For this review, take the finished solid that the model builds, in its own axes (mm). Face numbers are marked on the shaded views. A direction names the side the tool comes from. Coordinates: 2 decimals unless noted, no trailing zeros. Loops run counter-clockwise (first coordinate to the right, second up) from the corner with the lowest first, then second, coordinate; pieces in that order, holes last. Notation, with made-up numbers: (50.25, 5.5) - (54.25, 5.5) arc R22 ccw to (54.25, 35.5) - close; hole circle Ø7 at (86, 18.25). An arc over 180 degrees is marked (long way). Answer as a JSON object with one key per item and string values. Group by question number.
Item 1: We need section B-B (x = -16). Give the boundary of the cut face in (y, z).
Item 2: Clearance check with flat-ended pins moving along their axes: pin 1 (1.5 mm diameter, centred on y = 3.5, z = 4, fed in from -X); pin 2 (6.5 mm diameter, centred on x = 3.5, z = -4.5, fed in from +Y); pin 3 (3 mm diameter, centred on x = -2, z = 9.5, fed in from +Y); pin 4 (4 mm diameter, centred on x = 10.5, y = 5, fed in from +Z). State where each tip first meets the part, or that it passes through.
Item 3: We need section A-A (y = 4.5). Give the boundary of the cut face in (x, z), then the cut area to 3 significant figures.
Item 4: To check wall thickness, follow line 1 (X direction, y = 5, z = 8); line 2 (Z direction, x = 15, y = 3.25); line 3 (X direction, y = 6.25, z = -3). State the ranges of each line that lie inside material, in increasing order.
Item 5: We need section D-D (z = 8). Give the boundary of the cut face in (x, y), then the cut area to 3 significant figures.
Item 6: We need section C-C (z = 1). Give the boundary of the cut face in (x, y), then the cut area to 3 significant figures.
Item 7: Mouldability with a two-part tool opening along X and no side actions: class the marked faces 5, 6 and 7 as released by +X, released by -X, zero draft, split by the parting line, or undercut.
Item 8: Tool access review of the marked faces 1, 2, 3 and 4: name each direction out of +Z, -Z, +X, -X, +Y, -Y from which nothing blocks a thin tool from reaching the whole face with its end or side.
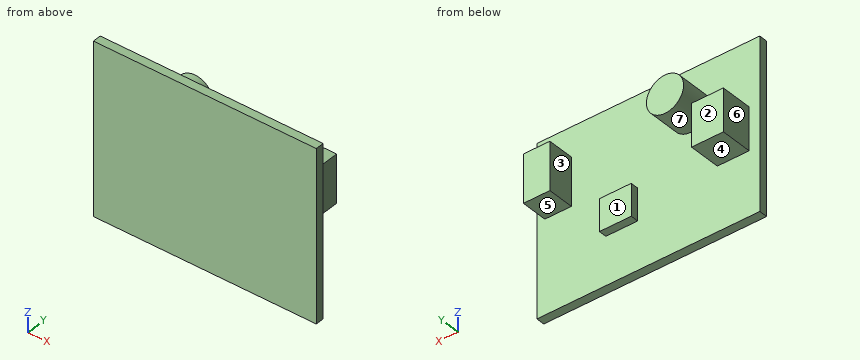
from build123d import *

# Parameters (mm, degrees)
SKETCH1_W             = 42
SKETCH1_H             = 32
PCB_DEPTH             = 1.6
IC_START              = 1.6
SKETCH2_W             = 6
SKETCH2_H             = 6
IC_DEPTH              = 1.5
OUT_CONNECTOR_START   = 1.6
SKETCH3_W             = 5
SKETCH3_H             = 9
OUT_CONNECTOR_DEPTH   = 5
PROBE_CONNECTOR_START = 1.6
SKETCH4_W             = 6
SKETCH4_H             = 8
PROBE_CONNECTOR_DEPTH = 6
TRIM_POT_START        = 1.6
SKETCH5_R             = 3.5
TRIM_POT_DEPTH        = 6


with BuildPart() as part:
    # Sketch1 → PCB (new body)
    with BuildSketch(Plane(origin=(0, 0, 0), x_dir=(1, 0, 0), z_dir=(0, 1, 0))):
        Rectangle(SKETCH1_W, SKETCH1_H)
    extrude(amount=PCB_DEPTH)

    # Sketch2 → IC (add)
    with BuildSketch(Plane(origin=(0, 0, 0), x_dir=(1, 0, 0), z_dir=(0, 1, 0)).offset(IC_START)):
        with Locations((5, 4)):
            Rectangle(SKETCH2_W, SKETCH2_H)
    extrude(amount=IC_DEPTH)

    # Sketch3 → Out_Connector (add)
    with BuildSketch(Plane(origin=(0, 0, 0), x_dir=(1, 0, 0), z_dir=(0, 1, 0)).offset(OUT_CONNECTOR_START)):
        with Locations((17, -6)):
            Rectangle(SKETCH3_W, SKETCH3_H)
    extrude(amount=OUT_CONNECTOR_DEPTH)

    # Sketch4 → Probe_Connector (add)
    with BuildSketch(Plane(origin=(0, 0, 0), x_dir=(1, 0, 0), z_dir=(0, 1, 0)).offset(PROBE_CONNECTOR_START)):
        with Locations((-16, 0)):
            Rectangle(SKETCH4_W, SKETCH4_H)
    extrude(amount=PROBE_CONNECTOR_DEPTH)

    # Sketch5 → Trim_Pot (add)
    with BuildSketch(Plane(origin=(0, 0, 0), x_dir=(1, 0, 0), z_dir=(0, 1, 0)).offset(TRIM_POT_START)):
        with Locations(Location((-8, -8, 0), (0, 0, 90))):
            Circle(SKETCH5_R)
    extrude(amount=TRIM_POT_DEPTH)


solid = part.part
Check sheet entries:
{
 "1": {"outline": "(0, -16) - (1.6, -16) - (1.6, -4) - (7.6, -4) - (7.6, 4) - (1.6, 4) - (1.6, 16) - (0, 16) - close"},
 "2": {"pin 1": "stops at x = -19", "pin 2": "stops at y = 3.1", "pin 3": "stops at y = 1.6", "pin 4": "passes through"},
 "3": {"outline": "(-19, -4) - (-13, -4) - (-13, 4) - (-19, 4) - close; circle Ø7 at (-8, 8); (14.5, 1.5) - (19.5, 1.5) - (19.5, 10.5) - (14.5, 10.5) - close", "area": "131 mm2"},
 "4": {"line 1": "x = -11.5 to -4.5, 14.5 to 19.5", "line 2": "z = 1.5 to 10.5", "line 3": "x = -19 to -13"},
 "5": {"outline": "(-21, 0) - (21, 0) - (21, 1.6) - (19.5, 1.6) - (19.5, 6.6) - (14.5, 6.6) - (14.5, 1.6) - (-4.5, 1.6) - (-4.5, 7.6) - (-11.5, 7.6) - (-11.5, 1.6) - (-21, 1.6) - close", "area": "134 mm2"},
 "6": {"outline": "(-21, 0) - (21, 0) - (21, 1.6) - (-13, 1.6) - (-13, 7.6) - (-19, 7.6) - (-19, 1.6) - (-21, 1.6) - close", "area": "103 mm2"},
 "7": {"face 5": "zero draft", "face 6": "released by -X", "face 7": "undercut"},
 "8": {"face 1": "+Z, -Z, +X, +Y", "face 2": "+Z, -Z, +X, -X, +Y", "face 3": "+Z, -Z, +Y", "face 4": "-Z, -X, +Y"}
}
